Input: part model. Units: mm. Frame: model coordinates. Face numbers are marked on the shaded views. A direction names the side the tool comes from. Coordinates: 2 decimals unless noted, no trailing zeros. Order: outer loops, then holes, each group sorted by start corner. A loop starts at its lowest first (then second) coordinate and runs counter-clockwise, first axis right, second up. Notation, with made-up numbers: M -27,32 L 29,32 A20 ccw 29,55 Z; hole C -4,69 d2. An arc over 180 degrees is marked long. Answer in a Markdown table with one row per item.
from build123d import *

# Parameters (mm, degrees)
F0_R      = 5.969
F1_DEPTH  = 115.316
F3_DEPTH  = 19.05
F1_FACE_R = 5.969
F5_ANGLE  = -180
F6_R      = 1.27
F7_W      = 13.208
F7_H      = 15.24
F8_DEPTH  = 21.844


with BuildPart() as f1:
    # F0 (on Top) → F1 (new body)
    with BuildSketch(Plane.XY):
        with Locations((7.493, 0)):
            Circle(F0_R)
        with Locations((-7.493, 0)):
            Circle(F0_R)
    extrude(amount=F1_DEPTH)

    # F2 (on Top) → F3 (join)
    with BuildSketch(Plane.XY):
        with BuildLine():
            ThreePointArc((-15.621, -0.508), (-13.165969, -6.434969), (-7.239, -8.89))
            Line((-7.239, -8.89), (7.239, -8.89))
            ThreePointArc((7.239, -8.89), (13.165969, -6.434969), (15.621, -0.508))
            Line((15.621, -0.508), (15.621, 0.508))
            ThreePointArc((15.621, 0.508), (13.165969, 6.434969), (7.239, 8.89))
            Line((7.239, 8.89), (-7.239, 8.89))
            ThreePointArc((-7.239, 8.89), (-13.165969, 6.434969), (-15.621, 0.508))
            Line((-15.621, 0.508), (-15.621, -0.508))
        make_face()
    extrude(amount=-F3_DEPTH)

    # F1_face (on face) → F5 (revolve)
    with BuildSketch(Plane(origin=(-7.493, 0, 115.316), x_dir=(1, 0, 0), z_dir=(0, 0, 1))):
        with Locations((14.986, 0)):
            Circle(F1_FACE_R)
    revolve(axis=Axis((0, 21.043353, 115.316), (0, 1, 0)), revolution_arc=F5_ANGLE)

    # F6
    f6_edges = [f1.edges().sort_by_distance(p)[0] for p in [
        (0, -8.89, 0),
    ]]
    fillet(f6_edges, radius=F6_R)

    # F7 (on face) → F8 (join)
    with BuildSketch(Plane(origin=(0, 0, -19.05), x_dir=(1, 0, 0), z_dir=(0, 0, -1))):
        Rectangle(F7_W, F7_H)
    extrude(amount=F8_DEPTH)


solid = f1.part
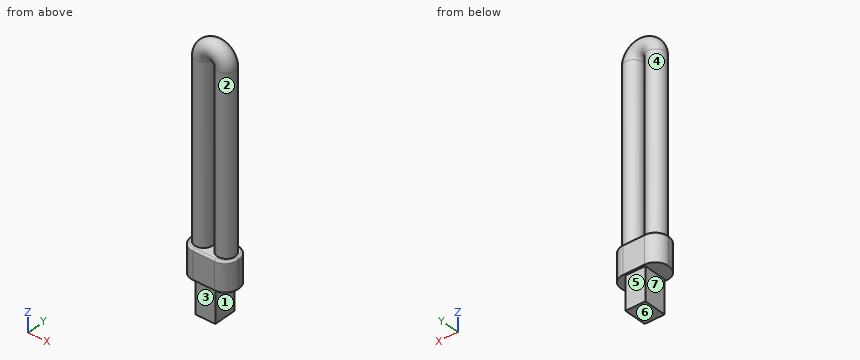
1) Material intervals for probe 1 along X at (y, z) = (-0.5, 77); probe 2 along X at (y, z) = (2, 113); probe 3 along Z at (x, y) = (-1, -7), sorted ascending.
Resolved:
| item | result |
|---|---|
| probe 1 | x = -13.44 to -1.54, 1.54 to 13.44 |
| probe 2 | x = -13.12 to -1.87, 1.87 to 13.12 |
| probe 3 | z = -40.89 to 0 |
2) Contact query for flat-ended pins moving along their axis: pin 1 (7.5 mm diameter, centred on y = 0, z = -30.5, fed in from +X); pin 2 (7.5 mm diameter, centred on x = -5, y = -2, fed in from +Z); pin 3 (2 mm diameter, centred on x = 5, y = 5.5, fed in from +Z). Output: stop coordinate, or through.
Resolved:
| item | result |
|---|---|
| pin 1 | stops at x = 6.6 |
| pin 2 | stops at z = 128.67 |
| pin 3 | stops at z = 125.66 |
3) Reachability of the marked faces 5, 6 and 7 from +Z, -Z, +X, -X, +Y, -Y: full face, straight path, thin tool, end or side. Return the list, or none.
Resolved:
| item | result |
|---|---|
| face 5 | -Z, +X, -X, +Y |
| face 6 | -Z, +X, -X, +Y, -Y |
| face 7 | -Z, -X, +Y, -Y |
4) Mould query, pull axis X, two halves, no side actions, for the marked faces 1, 2, 3 and 4. Classes: +X half, -X half, draft (parallel to the pull), parting line (faces both ways), or undercut.
Resolved:
| item | result |
|---|---|
| face 1 | +X half |
| face 2 | undercut |
| face 3 | draft |
| face 4 | undercut |
5) Cut plane A-A, the plane z = -16. Output: boundary loops of the cut face in (x, y), and give its area (3 significant figures).
Resolved:
| item | result |
|---|---|
| outline | M -15.62,-0.51 A8.38 ccw -7.24,-8.89 L 7.24,-8.89 A8.38 ccw 15.62,-0.51 L 15.62,0.51 A8.38 ccw 7.24,8.89 L -7.24,8.89 A8.38 ccw -15.62,0.51 Z |
| area | 495 mm2 |
6) Cut plane B-B, the plane z = 38.5. Output: boundary loops of the cut face in (x, y), and give its area (3 significant figures).
Resolved:
| item | result |
|---|---|
| outline | C -7.49,0 d11.94; C 7.49,0 d11.94 |
| area | 224 mm2 |
